Check sheet for the drawn part. Datum: minimum x, y, z corner. Units: mm. A direction names the side the tool comes from. Give positions to 0.01 mm unless a question says otherwise; leave off trailing zeros. Write each loop counter-clockwise with the first axis right and the second up, starting at its lowest first coordinate (ties: lowest second). Pieces come first, ordered by that corner, then holes. Notation, with made-up numbers: (35.5, 46.25) - (39.5, 46.25) arc R13 ccw to (39.5, 54.25) - close; hole circle Ø8 at (53, -16). An arc over 180 degrees is marked (long way). One line per question, with ' | ' between items. Start each with the question number.
Q1. Section check B-B on y = 37.5. Record the boundary of the cut face in (x, z).
Q2. Gauge pin test, flat ends, axial feed: P1, Ø11, axis at x = 63.5, y = 70.7, coming from the -Z side; P2, Ø6, axis at x = 88.9, z = 20.955, coming from the +Y side; P3, Ø12, axis at x = 96.5, z = 64.5, coming from the -Y side; P4, Ø8.5, axis at x = 63.5, y = 39.79, coming from the -Z side. Record the tip position at first contact, or that the pin passes through.
Q3. Set-up check for the marked faces 1 and 2: record each of +Z, -Z, +X, -X, +Y, -Y from which the full face is reachable in a straight line by a thin tool's end or side.
Q4. Thickness scan on L1, parallel to Y at x = 63.5, z = 97.25 (1 decimal); L2, parallel to Z at x = 88, y = 1; L3, parallel to Z at x = 72, y = 31. Record the ranges inside material, lowest first. Write a range as [from, to].
Q5. Section check A-A on x = 63.5. Count the separate pieces of the cut face and the enclosed holes in it, and give its area (3 significant figures).
Q6. Section check C-C on x = 88.9. Record the boundary of the cut face in (y, z).
Q7. Section check D-D on z = 58. Record the boundary of the cut face in (x, y).
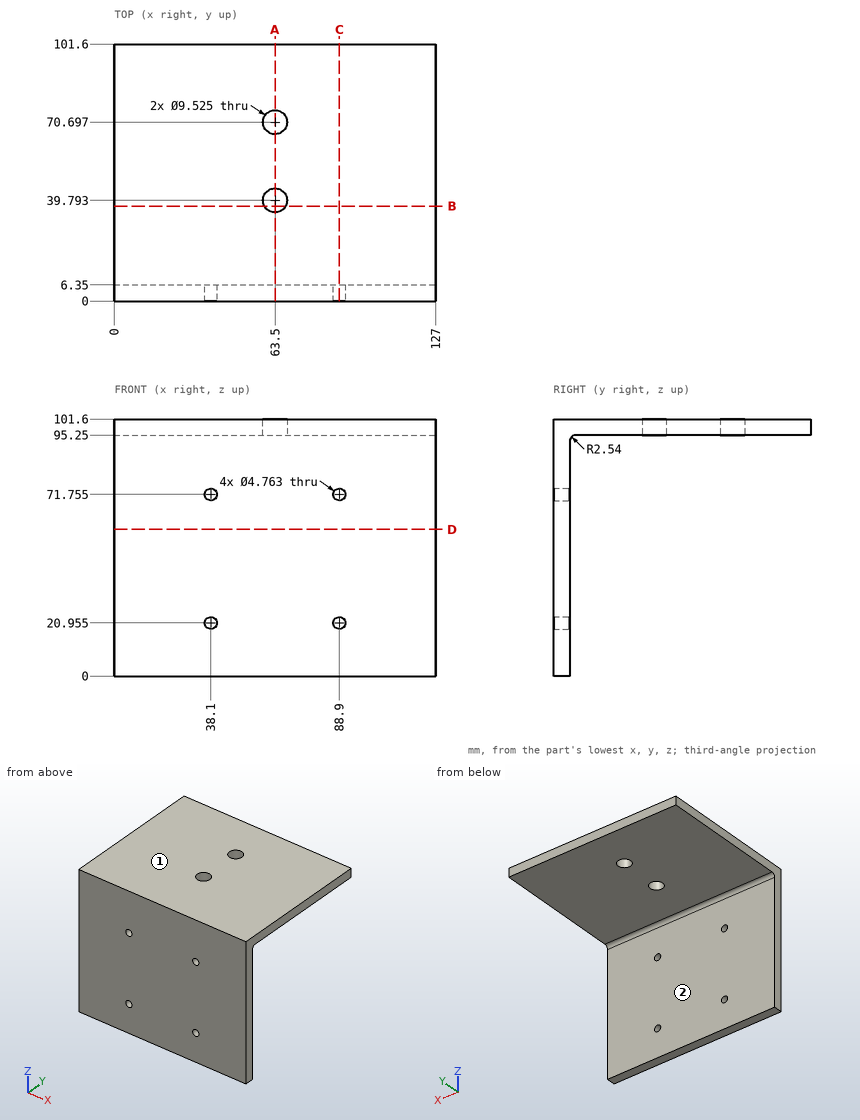
Working result:
1) outline: (0, 95.25) - (59.33, 95.25) - (59.33, 101.6) - (0, 101.6) - close; (67.67, 95.25) - (127, 95.25) - (127, 101.6) - (67.67, 101.6) - close
2) P1: stops at z = 95.25 | P2: stops at y = 6.35 | P3: stops at y = 0 | P4: passes through
3) face 1: +Z, +X, -X, +Y, -Y | face 2: -Z, +X, -X, +Y
4) L1: y = [0, 35], [44.6, 65.9], [75.5, 101.6] | L2: z = [0, 18.75], [23.16, 69.55], [73.96, 101.6] | L3: z = [95.25, 101.6]
5) separate pieces: 3 | enclosed holes: 0 | area: 1,130 mm2
6) outline: (0, 0) - (6.35, 0) - (6.35, 18.57) - (0, 18.57) - close; (0, 23.34) - (6.35, 23.34) - (6.35, 69.37) - (0, 69.37) - close; (0, 74.14) - (6.35, 74.14) - (6.35, 92.71) arc R2.54 cw to (8.89, 95.25) - (101.6, 95.25) - (101.6, 101.6) - (0, 101.6) - close
7) outline: (0, 0) - (127, 0) - (127, 6.35) - (0, 6.35) - close
